Geometry: see drawing. Coordinates: mm, zero at the bounding-box minimum. Round coordinates to 2 decimals unless told otherwise and drop trailing zeros. Order: outer loops, then holes, each group sorted by start corner. A loop starts at its lowest first (then second) coordinate and runs counter-clockwise, first axis right, second up. Notation, with made-up numbers: (86, 62) -> (133, 62) arc R9 cw to (133, 76) -> close; hole circle Ø11 at (-37.5, -20). An arc over 180 degrees is marked (long way). Answer as CSV lines item,"result". Start each with the question number.
(1) Section query C-C (z = 50). Output: boundary loops of the cut face in (x, y).
(2) Contact query for a flat-ended pin moving along its axis: P1, Ø6, axis at x = 74, z = 38, coming from the -Y side. Output: stop coordinate, or through.
(3) Pull-direction query (Z, two-part tool) for the marked faces 1, 2, 3 and 4; classes: +Z half, -Z half, draft (parallel to the pull), parting line (faces both ways), or undercut.
(4) Section query A-A (y = 9). Output: boundary loops of the cut face in (x, z), plus the area to 3 significant figures.
(5) Section query B-B (x = 99.5). Output: boundary loops of the cut face in (y, z).
(6) Section query D-D (x = 52.5). Output: boundary loops of the cut face in (y, z), plus the area to 3 significant figures.
(7) Line query: line 1 along Z through (x, y) = (99.5, 4.75); line 2 along X through (y, z) = (7.5, 85.5); line 3 along X through (y, z) = (9, 11.5). Output: solid intervals per line, ascending. Write a range as from..to.
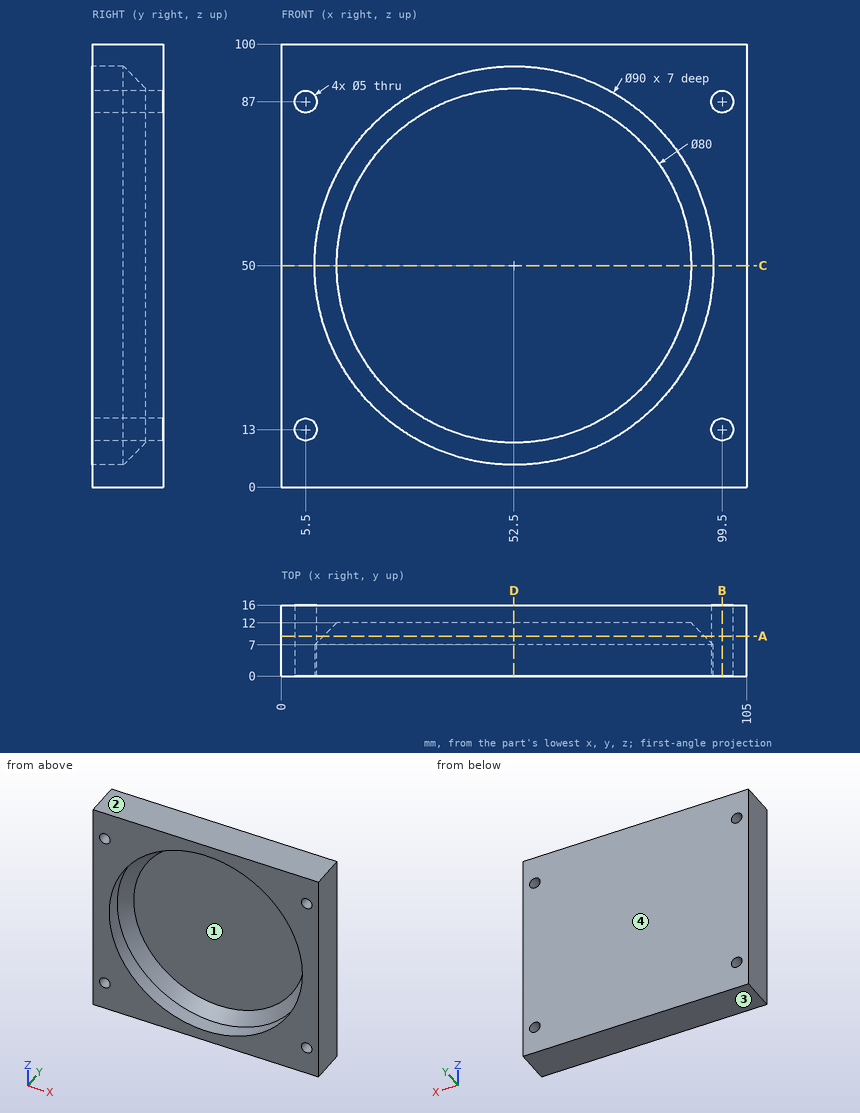
Answer block:
1,outline,"(0, 0) -> (7.5, 0) -> (7.5, 7) -> (12.5, 12) -> (92.5, 12) -> (97.5, 7) -> (97.5, 0) -> (105, 0) -> (105, 16) -> (0, 16) -> close"
2,P1,"y = 12"
3,face 1,"undercut"
3,face 2,"+Z half"
3,face 3,"-Z half"
3,face 4,"draft"
4,outline,"(0, 0) -> (105, 0) -> (105, 100) -> (0, 100) -> close; hole circle Ø5 at (5.5, 13); hole circle Ø5 at (5.5, 87); hole circle Ø86 at (52.5, 50); hole circle Ø5 at (99.5, 13); hole circle Ø5 at (99.5, 87)"
4,area,"4,610 mm2"
5,outline,"(0, 0) -> (16, 0) -> (16, 10.5) -> (0, 10.5) -> close; (0, 15.5) -> (16, 15.5) -> (16, 84.5) -> (0, 84.5) -> close; (0, 89.5) -> (16, 89.5) -> (16, 100) -> (0, 100) -> close"
6,outline,"(0, 0) -> (16, 0) -> (16, 100) -> (0, 100) -> (0, 95) -> (7, 95) -> (12, 90) -> (12, 10) -> (7, 5) -> (0, 5) -> close"
6,area,"545 mm2"
7,line 1,"0..10.5, 15.5..84.5, 89.5..100"
7,line 2,"0..3.5, 7.5..25.67, 79.33..97.5, 101.5..105"
7,line 3,"0..3.5, 7.5..33.35, 71.65..97.5, 101.5..105"
